Check sheet for the modelled part. Datum: model origin and axes. Units: mm. A direction names the side the tool comes from. Round coordinates to 2 decimals unless told otherwise and drop trailing zeros. Order: outer loops, then holes, each group sorted by start corner. A loop starts at its lowest first (then second) coordinate and runs counter-clockwise, first axis right, second up.
from build123d import *

# Parameters (mm, degrees)
F2_T     = -2.54
F3_R     = 3
F4_DEPTH = 140.001


with BuildPart() as f1:
    # F0 (on Front) → F1 (revolve)
    with BuildSketch(Plane.XZ):
        with BuildLine():
            Line((0, 242.5), (0, -242.5))
            Line((0, -242.5), (115, -242.5))
            ThreePointArc((115, -242.5), (122.0710678119, -239.5710678119), (125, -232.5))
            Line((125, -232.5), (125, 222.5))
            Line((125, 222.5), (140, 222.5))
            Line((140, 222.5), (140, 242.5))
            Line((140, 242.5), (0, 242.5))
        make_face()
    revolve(axis=Axis((0, 0, 0), (0, 0, -1)))

    # F2
    f2_openings = [f1.faces().sort_by_distance(p)[0] for p in [
        (0, 0, 242.5),
    ]]
    offset(amount=F2_T, openings=f2_openings, kind=Kind.INTERSECTION)

    # F3 (on Front) → F4 (cut, through all)
    with BuildSketch(Plane.XZ):
        with Locations((0, 160)):
            Circle(F3_R)
        with Locations((0, -40)):
            Circle(F3_R)
        with Locations((0, -190)):
            Circle(F3_R)
    extrude(amount=-F4_DEPTH, mode=Mode.SUBTRACT)


solid = f1.part
1) Draft check along Y on faces 1 (the face through (-111.1, 85.19, 232.64)), 2 (the face through (-109.084, 83.642, 233.892)), 3 (the face through (2, -2, -239.96)), 4 (the face through (53, -115, 222.5)). Enter one of: pulls with the +Y half, pulls with the -Y half, needs draft (parallel to the pull), parting line crosses it, or undercut.
2) Set-up check for faces 5 (the face through (93, 103, 242.5)), 6 (the face through (-26.547, 119.548, -0.527)), 7 (the face through (-124.88, -5.5, -1.81)): record each of +Z, -Z, +X, -X, +Y, -Y from which the full face is reachable in a straight line by a thin tool's end or side.
3) Scan lines: line 1 (Y direction, x = -5, z = -37); line 2 (Z direction, x = 0, y = 123.25); line 3 (Z direction, x = 0, y = 123.4). Record each from-to range of solid material in increasing order.
4) Gauge pin test, flat ends, axial feed: pin 1 (5 mm diameter, centred on x = 95.5, y = 18.5, fed in from +Z); pin 2 (10 mm diameter, centred on y = -71.5, z = -62.5, fed in from -X); pin 3 (5.5 mm diameter, centred on x = 0, z = 160, fed in from +Y). Record the tip position at first contact, or that the pin passes through.
5) Sectioned sample at A-A on y = 0. Record the cut outline in (x, z).
6) Sectioned sample at B-B on z = 144.5. Record the cut outline in (x, y).
Values found:
1. face 1: parting line crosses it
1. face 2: undercut
1. face 3: undercut
1. face 4: needs draft
2. face 5: +Z, +X, -X, +Y, -Y
2. face 6: +Z
2. face 7: -Z
3. line 1: y = -124.9 to -122.36, 122.36 to 124.9
3. line 2: z = -238.15 to -193, -187 to -43, -37 to 157, 163 to 225.04
3. line 3: z = -237.93 to -193, -187 to -43, -37 to 157, 163 to 225.04
4. pin 1: stops at z = -239.96
4. pin 2: stops at x = -105.84
4. pin 3: stops at y = -122.43
5. outline: (-140, 222.5) - (-125, 222.5) - (-125, -232.5) arc R10 ccw to (-115, -242.5) - (115, -242.5) arc R10 ccw to (125, -232.5) - (125, 222.5) - (140, 222.5) - (140, 242.5) - (137.46, 242.5) - (137.46, 225.04) - (122.46, 225.04) - (122.46, -232.5) arc R7.46 cw to (115, -239.96) - (-115, -239.96) arc R7.46 cw to (-122.46, -232.5) - (-122.46, 225.04) - (-137.46, 225.04) - (-137.46, 242.5) - (-140, 242.5) - close
6. outline: circle Ø250 at (0, 0); hole circle Ø244.92 at (0, 0)
